```python
from build123d import *

# Parameters (mm, degrees)
SKETCH1_R           = 1.6
BOSS_EXTRUDE1_DEPTH = 35


with BuildPart() as part:
    # Sketch1 → Boss-Extrude1 (new body)
    with BuildSketch(Plane(origin=(0, 0, 0), x_dir=(-1, 0, 0), z_dir=(0, 0, 1))):
        with BuildLine():
            ThreePointArc((6.106952435, -11.464428538), (9.097104038, -7.574548586), (13.577547372, -5.575098618))
            Line((13.577547372, -5.575098618), (17.094474376, -4.96453424))
            ThreePointArc((17.094474376, -4.96453424), (20.427458361, 3.094361133), (11.812394993, 1.739643439))
            Line((11.812394993, 1.739643439), (10.395840134, -1.536777892))
            ThreePointArc((10.395840134, -1.536777892), (7.403500619, -5.424975016), (2.921933136, -7.421904043))
            Line((2.921933136, -7.421904043), (-0.867040687, -8.0775021))
            ThreePointArc((-0.867040687, -8.0775021), (-3.926102771, -16.093293092), (4.58295671, -14.994806488))
            Line((4.58295671, -14.994806488), (6.106952435, -11.464428538))
        make_face()
        with Locations((0, -13)):
            Circle(SKETCH1_R, mode=Mode.SUBTRACT)
        with Locations((16.5, 0)):
            Circle(SKETCH1_R, mode=Mode.SUBTRACT)
    extrude(amount=BOSS_EXTRUDE1_DEPTH)


solid = part.part
```
Source: CAD feature listing. Evaluate the final solid. Frame: model axes, mm. Round coordinates to 2 decimals unless told otherwise and drop trailing zeros. Loops run counter-clockwise (first coordinate to the right, second up) from the corner with the lowest first, then second, coordinate; pieces in that order, holes last.
1. Contact query for flat-ended pins moving along their axis: pin 1 (1.5 mm diameter, centred on x = -7, z = 5.5, fed in from -Y); pin 2 (4 mm diameter, centred on y = 4.5, z = 30.5, fed in from +X); pin 3 (6 mm diameter, centred on x = -12.5, z = 20, fed in from -Y); pin 4 (3 mm diameter, centred on x = 0, y = 13, fed in from -Z). Output: stop coordinate, or through.
2. Section query A-A on y = 0.5. Output: boundary loops of the cut face in (x, z).
3. Mould query, pull axis Y, two halves, no side actions, for faces 1 (the cylindrical face through (-14.9, -0.07, 17.26)), 2 (the cylindrical face through (0.35, 14.56, 17.26)), 3 (the flat face through (-11.11, -0.12, 17.26)), 4 (the cylindrical face through (-20.5, -3, 17.3)). Classes: released by +Y, released by -Y, zero draft, split by the parting line, or undercut.
4. Ray query, L1, parallel to Y at x = -16.5, z = 23; L2, parallel to X at y = 0, z = 18.5; L3, parallel to Y at x = -0.75, z = 12.5. Return the intervals inside material, ascending.
5. Section query C-C on z = 8. Output: boundary loops of the cut face in (x, y).
6. Section query B-B on x = -16.5. Output: boundary loops of the cut face in (y, z), and give its area (3 significant figures).
7. Section query D-D on y = 8.5. Output: boundary loops of the cut face in (x, z).
Answers below:
1. pin 1: stops at y = 5.14
1. pin 2: stops at x = -5.71
1. pin 3: stops at y = -4.9
1. pin 4: passes through
2. outline: (-21.47, 0) - (-18.02, 0) - (-18.02, 35) - (-21.47, 35) - close; (-14.98, 0) - (-10.84, 0) - (-10.84, 35) - (-14.98, 35) - close
3. face 1: undercut
3. face 2: undercut
3. face 3: released by -Y
3. face 4: split by the parting line
4. L1: y = -5 to -1.6, 1.6 to 5.07
4. L2: x = -21.5 to -18.1, -14.9 to -11.06
4. L3: y = 7.8 to 11.59, 14.41 to 17.94
5. outline: (-17.09, 4.96) arc R5 ccw (long way) to (-11.81, -1.74) - (-10.4, 1.54) arc R10 cw to (-2.92, 7.42) - (0.87, 8.08) arc R5 ccw (long way) to (-4.58, 14.99) - (-6.11, 11.46) arc R10 cw to (-13.58, 5.58) - close; hole circle Ø3.2 at (-16.5, 0); hole circle Ø3.2 at (0, 13)
6. outline: (-5, 0) - (-1.6, 0) - (-1.6, 35) - (-5, 35) - close; (1.6, 0) - (5.07, 0) - (5.07, 35) - (1.6, 35) - close
6. area: 240 mm2
7. outline: (-8.08, 0) - (2.18, 0) - (2.18, 35) - (-8.08, 35) - close
